from build123d import *

# Parameters (mm, degrees)
EXTRUDE_1_DEPTH     = 5
SKETCH_5_R          = 5.25
CUT_EXTRUDE_1_DEPTH = 5
EXTRUDE_3_DEPTH     = 5
SKETCH_10_R         = 1.5
CUT_EXTRUDE_2_DEPTH = 36.864078478


with BuildPart() as part:
    # 草图1 → 凸台-拉伸1 (new body)
    with BuildSketch(Plane(origin=(0, 0, 0), x_dir=(0, 0, -1), z_dir=(1, 0, 0))):
        with BuildLine():
            Line((3.506544331, 7.190559565), (3.506544331, 32.190559565))
            Line((3.506544331, 32.190559565), (-3.506544331, 32.190559565))
            Line((-3.506544331, 32.190559565), (-3.506544331, 7.190559565))
            ThreePointArc((-3.506544331, 7.190559565), (0, -8), (3.506544331, 7.190559565))
        make_face()
    extrude(amount=EXTRUDE_1_DEPTH)

    # 草图5 → 切除-拉伸1 (cut)
    with BuildSketch(Plane(origin=(5, 0, 0), x_dir=(0, 0, -1), z_dir=(1, 0, 0))):
        Circle(SKETCH_5_R)
    extrude(amount=-CUT_EXTRUDE_1_DEPTH, mode=Mode.SUBTRACT)

    # 草图9 → 凸台-拉伸3 (add)
    with BuildSketch(Plane(origin=(5, 0, 0), x_dir=(0, 0, -1), z_dir=(1, 0, 0))):
        Polygon((-3.506544331, 32.190559565), (15, 32.190559565), (15, 26.190559565), (-15, 26.190559565), (-15, 32.190559565), align=None)
    extrude(amount=-EXTRUDE_3_DEPTH)

    # 草图10 → 切除-拉伸2 (cut, through all)
    with BuildSketch(Plane.ZY):
        with Locations((0, 29.190559565)):
            Circle(SKETCH_10_R)
        with Locations((-10, 29.190559565)):
            Circle(SKETCH_10_R)
        with Locations((10, 29.190559565)):
            Circle(SKETCH_10_R)
    extrude(amount=-CUT_EXTRUDE_2_DEPTH, mode=Mode.SUBTRACT)


solid = part.part
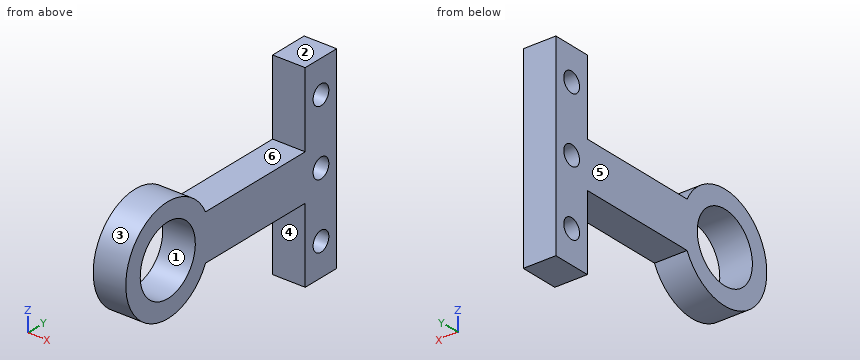
Verification items for the finished model (mm, model axes). Face numbers are marked on the shaded views. A direction names the side the tool comes from. Coordinates: 2 decimals unless noted, no trailing zeros. Order: outer loops, then holes, each group sorted by start corner. A loop starts at its lowest first (then second) coordinate and runs counter-clockwise, first axis right, second up.
Item 1: Section check A-A, the plane z = 0. Enter the section's corners in (x, y), then the cut area to 3 significant figures.
Filled in:
outline: (0, -8) - (5, -8) - (5, -5.25) - (0, -5.25) - close; (0, 5.25) - (5, 5.25) - (5, 27.69) - (0, 27.69) - close; (0, 30.69) - (5, 30.69) - (5, 32.19) - (0, 32.19) - close
area: 133 mm2
Item 2: Section check C-C, the plane z = -10. Enter the section's corners in (x, y).
Filled in:
outline: (0, 26.19) - (5, 26.19) - (5, 27.69) - (0, 27.69) - close; (0, 30.69) - (5, 30.69) - (5, 32.19) - (0, 32.19) - close
Item 3: Section check D-D, the plane x = 4.5. Enter the section's corners in (y, z), then the cut area to 3 significant figures.
Filled in:
outline: (7.19, -3.51) - (26.19, -3.51) - (26.19, -15) - (32.19, -15) - (32.19, 15) - (26.19, 15) - (26.19, 3.51) - (7.19, 3.51) arc R8 ccw (long way) to start; hole circle Ø10.5 at (0, 0); hole circle Ø3 at (29.19, -10); hole circle Ø3 at (29.19, 0); hole circle Ø3 at (29.19, 10)
area: 403 mm2
Item 4: Material ranges on L1, parallel to Y at x = 2.3, z = 0; L2, parallel to Z at x = 3.05, y = 30.5; L3, parallel to Y at x = 3.55, z = -10, recorded low to high.
Filled in:
L1: y = -8 to -5.25, 5.25 to 27.69, 30.69 to 32.19
L2: z = -15 to -10.73, -9.27 to -0.73, 0.73 to 9.27, 10.73 to 15
L3: y = 26.19 to 27.69, 30.69 to 32.19
Item 5: Release check for a two-part mould opening along Z. For the marked faces 1, 2 and 3 record: +Z half, -Z half, draft (parallel to the pull), parting line (faces both ways), or undercut.
Filled in:
face 1: undercut
face 2: +Z half
face 3: parting line
Item 6: Depth check by flat-ended pin: pin 1 (1.5 mm diameter, centred on x = 4.5, y = -3, fed in from +Z). Enter the tip coordinate at first touch or a pass-through.
Filled in:
pin 1: stops at z = 7.68
Item 7: Section check B-B, the plane y = 0. Enter the section's corners in (x, z), then the cut area to 3 significant figures.
Filled in:
outline: (0, -8) - (5, -8) - (5, -5.25) - (0, -5.25) - close; (0, 5.25) - (5, 5.25) - (5, 8) - (0, 8) - close
area: 27.5 mm2
Item 8: Access from +Z, -Z, +X, -X, +Y, -Y to the whole of each face (thin tool, end or side, straight path). Record for the marked faces 4, 5 and 6.
Filled in:
face 4: -Z, +X, -X
face 5: +Z, -Z, -X, +Y, -Y
face 6: +Z, +X, -X
